The drawing under review shows one solid part. Ordinate dimensions are in mm from its lowest x, y, z. Give positions to 0.01 mm unless a question says otherwise; leave off trailing zeros. Order: outer loops, then holes, each group sorted by start corner. A loop starts at its lowest first (then second) coordinate and runs counter-clockwise, first axis right, second up. Notation, with made-up numbers: (43, 60) -> (79, 60) arc R21 ccw to (79, 73) -> close; hole circle Ø6 at (47, 65.5). An arc over 180 degrees is marked (long way). Return JSON: item names as keys, results as strings. Group by question number.
1) Add section D-D (z = 26). Give the boundary of the cut face in (x, y).
2) Add section B-B (z = 5). Give the boundary of the cut face in (x, y) (1 decimal).
3) To check wall thickness, follow line 1 along Z through (x, y) = (57.15, 1.15) (1 decimal); line 2 along X through (y, z) = (0.45, 5) (1 decimal); line 3 along Z through (x, y) = (6.5, 1.3) (1 decimal). State the ranges of each line that lie inside material, in increasing order.
4) Add section C-C (x = 34). Give the boundary of the cut face in (y, z).
5) Add section A-A (y = 0.7). State how many separate pieces and enclosed holes the cut face has, then the cut area to 3 significant figures.
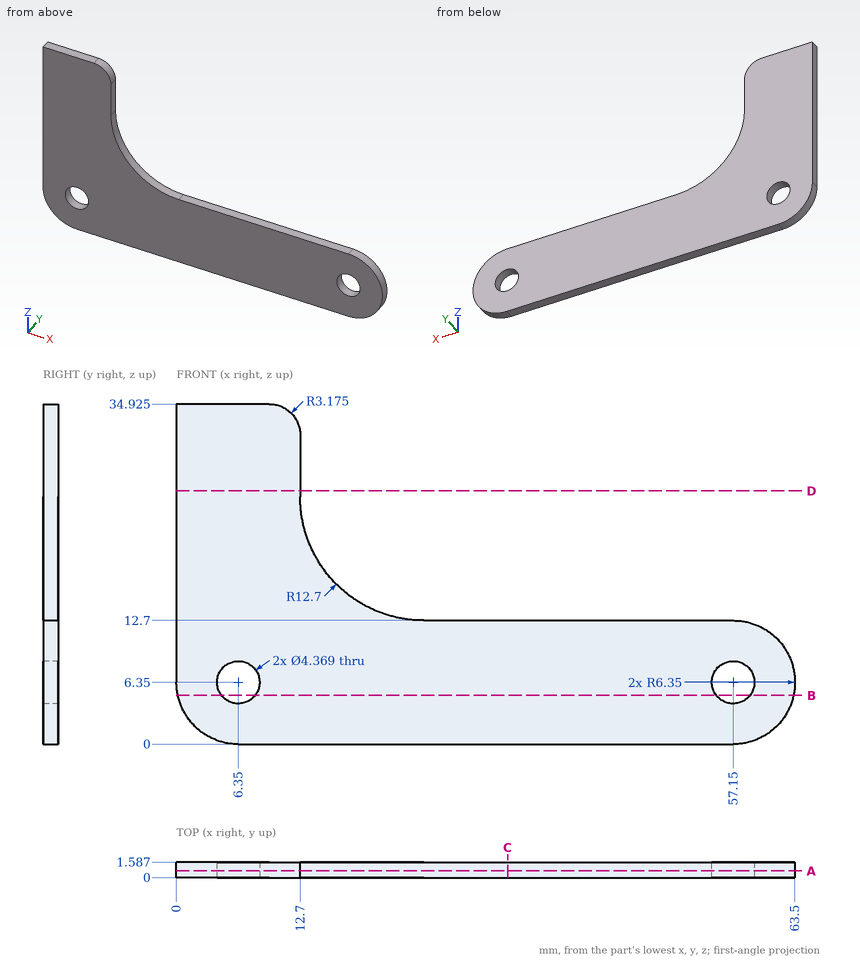
Evaluation:
{
 "1": {"outline": "(0, 0) -> (12.7, 0) -> (12.7, 1.59) -> (0, 1.59) -> close"},
 "2": {"outline": "(0.1, 0) -> (4.6, 0) -> (4.6, 1.6) -> (0.1, 1.6) -> close; (8.1, 0) -> (55.4, 0) -> (55.4, 1.6) -> (8.1, 1.6) -> close; (58.9, 0) -> (63.4, 0) -> (63.4, 1.6) -> (58.9, 1.6) -> close"},
 "3": {"line 1": "0 to 4.2, 8.5 to 12.7", "line 2": "0.1 to 4.6, 8.1 to 55.4, 58.9 to 63.4", "line 3": "0 to 4.2, 8.5 to 34.9"},
 "4": {"outline": "(0, 0) -> (1.59, 0) -> (1.59, 12.7) -> (0, 12.7) -> close"},
 "5": {"separate pieces": "1", "enclosed holes": "2", "area": "1,070 mm^2"}
}
